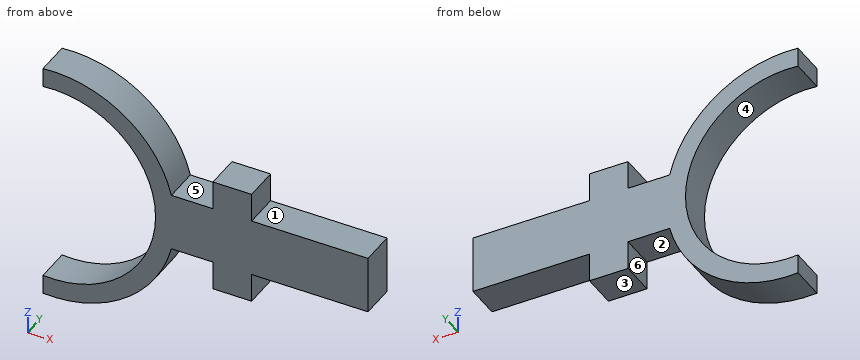
from build123d import *

# Parameters (mm, degrees)
SKETCH_1_R           = 6.326152672
SKETCH_1_R_2         = 5.326152672
EXTRUDE_1_DEPTH      = 1.8
EXTRUDE_2_DEPTH      = 10
EXTRUDE_2_DEPTH_BACK = 0.5
SKETCH_2_W           = 3
SKETCH_2_H           = 1.8
CUT_EXTRUDE_1_REACH  = 19.601
SKETCH_3_W           = 6.461960394
SKETCH_3_H           = 15
EXTRUDE_START        = -1.8
SKETCH_4_W           = 2
SKETCH_4_H           = 6
EXTRUDE_3_DEPTH      = 1.8


with BuildPart() as part:
    # 草图1 → 凸台-拉伸1 (new body)
    with BuildSketch(Plane(origin=(0, 0, 0), x_dir=(1, 0, 0), z_dir=(0, 1, 0))):
        with Locations(Location((0, 0, 0), (0, 0, 270))):
            Circle(SKETCH_1_R)
        with Locations(Location((0, 0, 0), (0, 0, 270))):
            Circle(SKETCH_1_R_2, mode=Mode.SUBTRACT)
    extrude(amount=EXTRUDE_1_DEPTH)

    # 草图2 → 凸台-拉伸2 (add, two sides: drawn at the far end of the back side and taken through both)
    with BuildSketch(Plane(origin=(6.326152672, 0, 0), x_dir=(0, 0, -1), z_dir=(1, 0, 0)).offset(-EXTRUDE_2_DEPTH_BACK)):
        with Locations((0, 0.9)):
            Rectangle(SKETCH_2_W, SKETCH_2_H)
    extrude(amount=EXTRUDE_2_DEPTH + EXTRUDE_2_DEPTH_BACK)

    # 草图3 → 切除-拉伸1 (cut, up to next)
    with BuildSketch(Plane(origin=(0, 1.8, 0), x_dir=(1, 0, 0), z_dir=(0, 1, 0)), mode=Mode.PRIVATE) as cut_extrude_1_sk1:
        with Locations((-3.730980197, 0.039566398)):
            Rectangle(SKETCH_3_W, SKETCH_3_H)
    cut_extrude_1_tool1 = extrude(cut_extrude_1_sk1.sketch, amount=-CUT_EXTRUDE_1_REACH, mode=Mode.PRIVATE) & part.part
    add(cut_extrude_1_tool1.solids().sort_by_distance((-3.73098, 1.8, -0.039566))[0], mode=Mode.SUBTRACT)

    # 草图4 → 凸台-拉伸3 (add)
    with BuildSketch(Plane(origin=(0, 1.8, 0), x_dir=(1, 0, 0), z_dir=(0, 1, 0)).offset(EXTRUDE_START)):
        with Locations((9.3, 0)):
            Rectangle(SKETCH_4_W, SKETCH_4_H)
    extrude(amount=EXTRUDE_3_DEPTH)


solid = part.part
Read the model definition and answer for the solid it produces. Units are mm, in the model's axes. Face numbers are marked on the shaded views. A direction names the side the tool comes from. Round coordinates to 2 decimals unless told otherwise and drop trailing zeros. Write each loop counter-clockwise with the first axis right and the second up, starting at its lowest first coordinate (ties: lowest second). Pieces come first, ordered by that corner, then holes.
1. Given pin 1 Ø0.9 at (x, y) = (13, 1) entering from -Z; pin 2 Ø0.8 at (y, z) = (1, -2) entering from -X; pin 3 Ø0.5 at (x, y) = (13.5, 1.5) entering from +Z, each flat-ended and moving along its own axis, determine where each tip first touches the part or whether it passes through.
2. The part is cut by section D-D, the plane x = 3.75. Determine the outline of the cut face in (y, z), then the cut area to 3 significant figures.
3. Determine the mould class of the marked faces 4, 5 and 6 for opening direction Z: pulls with the +Z half, pulls with the -Z half, needs draft (parallel to the pull), parting line crosses it, or undercut.
4. The part is cut by section A-A, the plane x = 0. Determine the outline of the cut face in (y, z), then the cut area to 3 significant figures.
5. Which of the six approach directions +Z, -Z, +X, -X, +Y, -Y give full straight-line access (tool end or side, diameter ignored) to the marked faces 1, 2 and 3?
6. The part is cut by section C-C, the plane z = -0.5. Determine the outline of the cut face in (x, y).
7. Straight lines are drawn through the part: L1, parallel to Z at x = 0, y = 0.85; L2, parallel to X at y = 1.2, z = 0; L3, parallel to Z at x = 7, y = 1.6. For each, find the intervals that lie inside material, in ascending order.
8. The part is cut by section B-B, the plane y = 0.3. Determine the outline of the cut face in (x, z), then the cut area to 3 significant figures.
Values:
1. pin 1: stops at z = -1.5
1. pin 2: stops at x = 4.75
1. pin 3: stops at z = 1.5
2. outline: (0, -5.09) - (1.8, -5.09) - (1.8, -3.78) - (0, -3.78) - close; (0, 3.78) - (1.8, 3.78) - (1.8, 5.09) - (0, 5.09) - close
2. area: 4.73 mm2
3. face 4: undercut
3. face 5: pulls with the +Z half
3. face 6: needs draft
4. outline: (0, -6.33) - (1.8, -6.33) - (1.8, -5.33) - (0, -5.33) - close; (0, 5.33) - (1.8, 5.33) - (1.8, 6.33) - (0, 6.33) - close
4. area: 3.60 mm2
5. face 1: +Z, +X, +Y, -Y
5. face 2: -Z, +Y, -Y
5. face 3: -Z, +X, +Y, -Y
6. outline: (5.3, 0) - (16.33, 0) - (16.33, 1.8) - (5.3, 1.8) - close
7. L1: z = -6.33 to -5.33, 5.33 to 6.33
7. L2: x = 5.33 to 16.33
7. L3: z = -1.5 to 1.5
8. outline: (-0.5, -6.31) arc R6.33 ccw to (6.15, -1.5) - (8.3, -1.5) - (8.3, -3) - (10.3, -3) - (10.3, -1.5) - (16.33, -1.5) - (16.33, 1.5) - (10.3, 1.5) - (10.3, 3) - (8.3, 3) - (8.3, 1.5) - (6.15, 1.5) arc R6.33 ccw to (-0.5, 6.31) - (-0.5, 5.3) arc R5.33 cw (long way) to (-0.5, -5.3) - close
8. area: 55.5 mm2
